from build123d import *

# Parameters (mm, degrees)
SKETCH1_R               = 6
BOSS_EXTRUDE1_DEPTH     = 20
SKETCH2_R               = 3.4
CUT_EXTRUDE1_DEPTH      = 13.55
SKETCH5_W               = 8.287891014
SKETCH5_H               = 8.876063753
BOSS_EXTRUDE2_DEPTH     = 18.26
SKETCH8_R               = 2.1
CUT_EXTRUDE6_DEPTH      = 30
CUT_EXTRUDE6_DEPTH_BACK = 30


with BuildPart() as part:
    # Sketch1 → Boss-Extrude1 (new body)
    with BuildSketch(Plane(origin=(0, 0, 0), x_dir=(1, 0, 0), z_dir=(0, 1, 0))):
        Circle(SKETCH1_R)
    extrude(amount=BOSS_EXTRUDE1_DEPTH)

    # Sketch2 → Cut-Extrude1 (cut)
    with BuildSketch(Plane(origin=(0, 20, 0), x_dir=(1, 0, 0), z_dir=(0, 1, 0))):
        Circle(SKETCH2_R)
    extrude(amount=-CUT_EXTRUDE1_DEPTH, mode=Mode.SUBTRACT)

    # Sketch5 → Boss-Extrude2 (add)
    with BuildSketch(Plane(origin=(0, 18.26, 0), x_dir=(1, 0, 0), z_dir=(0, 1, 0))):
        with Locations((6.743945507, -0.04378733)):
            Rectangle(SKETCH5_W, SKETCH5_H)
    extrude(amount=-BOSS_EXTRUDE2_DEPTH)

    # Sketch8 → Cut-Extrude6 (cut, two sides)
    with BuildSketch(Plane(origin=(0, 18.26, 0), x_dir=(1, 0, 0), z_dir=(0, 1, 0))) as cut_extrude6_sk:
        with Locations((4.580522752, 0)):
            Circle(SKETCH8_R)
    extrude(amount=CUT_EXTRUDE6_DEPTH, mode=Mode.SUBTRACT)
    extrude(cut_extrude6_sk.sketch, amount=-CUT_EXTRUDE6_DEPTH_BACK, mode=Mode.SUBTRACT)


solid = part.part
Model file for the job. Use its own axes, mm. A direction names the side the tool comes from. Give positions to 0.01 mm unless a question says otherwise; leave off trailing zeros. Loops run counter-clockwise (first coordinate to the right, second up) from the corner with the lowest first, then second, coordinate; pieces in that order, holes last. Notation, with made-up numbers: (38, 30) -> (58, 30) arc R18 ccw to (58, 48) -> close; hole circle Ø2 at (3.5, 85.5). An arc over 180 degrees is marked (long way). Use a Markdown table: item, result. Add a question column.
(1) Slice it at C-C on x = 0. List the corners of the cut face in (y, z), and give its area (3 significant figures).
(2) Drop flat-ended pins along their axis: pin 1 Ø3 at (x, z) = (-0.5, 0) entering from +Y; pin 2 Ø4 at (x, z) = (4.58, 0) entering from +Y; pin 3 Ø5.5 at (x, y) = (8.5, 9.5) entering from +Z; pin 4 Ø3 at (x, z) = (0.5, -2) entering from +Y. Give the stop position or say it passes through.
(3) Tool access for faces 4 (the flat face through (7, 9, -4.394)), 5 (the cylindrical face through (-3.4, 13.3, -0.1)), 6 (the cylindrical face through (6.584, 10.14, -0.631)): list every direction of +Z, -Z, +X, -X, +Y, -Y with a clear straight run to the whole face (end or side of a thin tool).
(4) Slice it at A-A on z = 0. List the corners of the cut face in (x, y), and give its area (3 significant figures).
(5) Mould opens along Z. For faces 1 (the cylindrical face through (-6, 10, 0)), 2 (the flat face through (7, 9, 4.482)), 3 (the flat face through (2.6, 12.4, -1.4)) say: +Z half, -Z half, draft (parallel to the pull), parting line (faces both ways), or undercut.
(6) Slice it at B-B on y = 10. List the corners of the cut face in (x, z), and give its area (3 significant figures).
(7) Wall check: line 1 along X through (y, z) = (5.5, 0); line 2 along Z through (x, y) = (0, 11.5); line 3 along X through (y, z) = (14.25, -1.5). Give the ranges that are in metal, low to high.
(8) Slice it at D-D on y = 2. List the corners of the cut face in (x, z), and give its area (3 significant figures).
Filled sheet:
| question | item | result |
|---|---|---|
| 1 | outline | (0, -6) -> (20, -6) -> (20, -3.4) -> (6.45, -3.4) -> (6.45, 3.4) -> (20, 3.4) -> (20, 6) -> (0, 6) -> close |
| 1 | area | 148 mm2 |
| 2 | pin 1 | y = 6.45 |
| 2 | pin 2 | through |
| 2 | pin 3 | z = 4.48 |
| 2 | pin 4 | y = 20 |
| 3 | face 4 | -Z, +X, +Y, -Y |
| 3 | face 5 | +Y |
| 3 | face 6 | +Y, -Y |
| 4 | outline | (-6, 0) -> (2.48, 0) -> (2.48, 6.45) -> (-3.4, 6.45) -> (-3.4, 20) -> (-6, 20) -> close; (6.68, 0) -> (10.89, 0) -> (10.89, 18.26) -> (6.68, 18.26) -> close |
| 4 | area | 167 mm2 |
| 5 | face 1 | parting line |
| 5 | face 2 | +Z half |
| 5 | face 3 | undercut |
| 6 | outline | (3.99, 4.48) arc R6 ccw (long way) to (4.09, -4.39) -> (10.89, -4.39) -> (10.89, 4.48) -> close; hole (2.6, -2.19) -> (2.6, -0.7) arc R2.1 ccw (long way) to (2.6, 0.7) -> (2.6, 2.19) arc R3.4 ccw (long way) to start |
| 6 | area | 114 mm2 |
| 7 | line 1 | -6 to 2.48, 6.68 to 10.89 |
| 7 | line 2 | -6 to -3.4, 3.4 to 6 |
| 7 | line 3 | -5.81 to -3.05, 2.6 to 3.11, 6.05 to 10.89 |
| 8 | outline | (3.99, 4.48) arc R6 ccw (long way) to (4.09, -4.39) -> (10.89, -4.39) -> (10.89, 4.48) -> close; hole circle Ø4.2 at (4.58, 0) |
| 8 | area | 148 mm2 |
